Can you work these out from the model? Positions are in its coordinate system, mm. A direction names the side the tool comes from. Round coordinates to 2 decimals unless told otherwise and drop trailing zeros. Write each loop counter-clockwise with the first axis right and the second up, starting at its lowest first coordinate (ties: lowest second). Pieces come first, ordered by that corner, then holes. Notation, with made-up numbers: M 89,55 L 122,55 A18 ccw 122,82 Z; hole C 2.25,67.5 d6. An arc over 180 degrees is marked long. Answer as a JSON object with one key per item and string values. Group by question number.
1) I'm going to push flat-ended pins straight in: pin 1 Ø8.5 at (x, z) = (58.74, 0) entering from +Y; pin 2 Ø12 at (x, z) = (-11.5, -27) entering from -Y; pin 3 Ø12.5 at (x, y) = (58.5, 41) entering from -Z. Where does each tip first touch, or does it pass through?
2) Suppose I cut it at C-C, the plane y = 31. Write out the boundary of the cut face in (x, z).
3) If we mould it in two halves opening along Z, with no side actions, what happens to faces 1 (the flat face through (-57.3, 18.359, -3.3)), 2 (the cylindrical face through (55.515, 9.051, -1.015)), 3 (the flat face through (42, 79, -88.9)), 4 (the flat face through (12.7, 79, -82))? For each: +Z half, -Z half, draft (parallel to the pull), parting line (faces both ways), or undercut.
4) On a 3-axis mill with a long thin cutter (end or side, diameter ignored), from which of +Z, -Z, +X, -X, +Y, -Y can I reach the whole of each face in a straight line? I mean faces 5 (the flat face through (-12.7, 79, -83)), 6 (the flat face through (-44.45, 38, 0)), 7 (the cylindrical face through (-65.874, 50.904, -0.314)). Say none if no direction works.
5) Suppose I cut it at D-D, the plane x = -49. Write out the boundary of the cut face in (y, z), and give its area (3 significant figures).
6) Suppose I cut it at A-A, the plane y = 12.5. Write out the boundary of the cut face in (x, z), and give its area (3 significant figures).
7) Suppose I cut it at B-B, the plane z = 0. Write out the boundary of the cut face in (x, y), and give its area (3 significant figures).
8) Please list where these lines run through material, in increasing order: L1, parallel to X at y = 15, z = -4; L2, parallel to Y at x = 41, z = 8; L3, parallel to Z at x = 46, y = 62.5. Write a range as [from, to].
from build123d import *

# Parameters (mm, degrees)
BOSS_EXTRUDE1_DEPTH                                  = 69.85
SKETCH2_W                                            = 88.9
SKETCH2_H                                            = 76.2
CUT_EXTRUDE1_DEPTH                                   = 149.378182358
CBORE_FOR_1_4_BINDING_HEAD_MACHINE_SCREW_D           = 6.7564
CBORE_FOR_1_4_BINDING_HEAD_MACHINE_SCREW_CBORE_D     = 14.2875
CBORE_FOR_1_4_BINDING_HEAD_MACHINE_SCREW_CBORE_DEPTH = 64.191007
CUT_EXTRUDE2_DEPTH                                   = 140.9883388


with BuildPart() as part:
    # Sketch1 → Boss-Extrude1 (new, symmetric)
    with BuildSketch(Plane(origin=(0, 0, 0), x_dir=(0, 0, -1), z_dir=(1, 0, 0))):
        Polygon((-12.7, 0), (12.7, 0), (12.7, 76.2), (88.9, 76.2), (88.9, 82.55), (-12.7, 82.55), align=None)
    extrude(amount=BOSS_EXTRUDE1_DEPTH, both=True)

    # Sketch2 → Cut-Extrude1 (cut, through all)
    with BuildSketch(Plane(origin=(0, 0, -88.9), x_dir=(-1, 0, 0), z_dir=(0, 0, -1))):
        with Locations((0, 38.1)):
            Rectangle(SKETCH2_W, SKETCH2_H)
    extrude(amount=-CUT_EXTRUDE1_DEPTH, mode=Mode.SUBTRACT)

    # CBORE for 1/4 Binding Head Machine Screw1 (through all)
    with Locations(Plane(origin=(0, 82.55, 0), x_dir=(1, 0, 0), z_dir=(0, 1, 0))):
        with Locations((58.7375, 0), (-58.7375, 0)):
            CounterBoreHole(CBORE_FOR_1_4_BINDING_HEAD_MACHINE_SCREW_D / 2, CBORE_FOR_1_4_BINDING_HEAD_MACHINE_SCREW_CBORE_D / 2, CBORE_FOR_1_4_BINDING_HEAD_MACHINE_SCREW_CBORE_DEPTH)

    # Sketch6 → Cut-Extrude2 (cut, through all)
    with BuildSketch(Plane(origin=(0, 82.55, 0), x_dir=(1, 0, 0), z_dir=(0, 1, 0))):
        with BuildLine():
            Line((12.7, 76.2), (12.7, 88.9))
            Line((12.7, 88.9), (-12.7, 88.9))
            Line((-12.7, 88.9), (-12.7, 76.2))
            ThreePointArc((-12.7, 76.2), (0, 63.5), (12.7, 76.2))
        make_face()
    extrude(amount=-CUT_EXTRUDE2_DEPTH, mode=Mode.SUBTRACT)


solid = part.part
Results:
{
 "1": {"pin 1": "y = 18.36", "pin 2": "y = 76.2", "pin 3": "z = -12.7"},
 "2": {"outline": "M -69.85,-12.7 L -44.45,-12.7 L -44.45,12.7 L -69.85,12.7 Z; M 44.45,-12.7 L 69.85,-12.7 L 69.85,12.7 L 44.45,12.7 Z; hole C -58.74,0 d14.29; hole C 58.74,0 d14.29"},
 "3": {"face 1": "undercut", "face 2": "undercut", "face 3": "-Z half", "face 4": "draft"},
 "4": {"face 5": "-Z, +Y, -Y", "face 6": "+Z, -Z, -Y", "face 7": "+Y"},
 "5": {"outline": "M 0,-12.7 L 76.2,-12.7 L 76.2,-88.9 L 82.55,-88.9 L 82.55,12.7 L 0,12.7 Z", "area": "2,580 mm^2"},
 "6": {"outline": "M -69.85,-12.7 L -44.45,-12.7 L -44.45,12.7 L -69.85,12.7 Z; M 44.45,-12.7 L 69.85,-12.7 L 69.85,12.7 L 44.45,12.7 Z; hole C -58.74,0 d6.76; hole C 58.74,0 d6.76", "area": "1,220 mm^2"},
 "7": {"outline": "M -69.85,0 L -62.12,0 L -62.12,18.36 L -65.88,18.36 L -65.88,82.55 L -69.85,82.55 Z; M -55.36,0 L -44.45,0 L -44.45,76.2 L 44.45,76.2 L 44.45,0 L 55.36,0 L 55.36,18.36 L 51.59,18.36 L 51.59,82.55 L -51.59,82.55 L -51.59,18.36 L -55.36,18.36 Z; M 62.12,0 L 69.85,0 L 69.85,82.55 L 65.88,82.55 L 65.88,18.36 L 62.12,18.36 Z", "area": "2,680 mm^2"},
 "8": {"L1": "[-69.85, -44.45], [44.45, 69.85]", "L2": "[76.2, 82.55]", "L3": "[-12.7, 12.7]"}
}
